```python
from build123d import *

# Parameters (mm, degrees)
SKETCH1_W              = 38.1
SKETCH1_H              = 76.2
BOSS_EXTRUDE1_DEPTH    = 2.54
F_1_0MM_DOWEL_HOLE1_D  = 19
M1_6_CLEARANCE_HOLE1_D = 1.8
M2_CLEARANCE_HOLE4_D   = 2.4
SKETCH15_R             = 3.749999993
BOSS_EXTRUDE2_DEPTH    = 10.000000066


with BuildPart() as part:
    # Sketch1 → Boss-Extrude1 (new body)
    with BuildSketch(Plane(origin=(0, 0, 0), x_dir=(1, 0, 0), z_dir=(0, 1, 0))):
        Rectangle(SKETCH1_W, SKETCH1_H)
    extrude(amount=BOSS_EXTRUDE1_DEPTH)

    # Ø1.0mm Dowel Hole1 (through all)
    with Locations(Plane(origin=(0, 2.54, 0), x_dir=(1, 0, 0), z_dir=(0, 1, 0))):
        with Locations((0, -13.000000035), (0, 13.000000035)):
            Hole(F_1_0MM_DOWEL_HOLE1_D / 2)

    # M1.6 Clearance Hole1 (through all)
    with Locations(Plane(origin=(0, 2.54, 0), x_dir=(1, 0, 0), z_dir=(0, 1, 0))):
        with Locations((8.750000026, 21.250000045), (8.750000026, -21.250000045), (-8.750000026, -21.250000045), (-8.750000026, 21.250000045)):
            Hole(M1_6_CLEARANCE_HOLE1_D / 2)

    # M2 Clearance Hole4 (through all)
    with Locations(Plane(origin=(0, 2.54, 0), x_dir=(1, 0, 0), z_dir=(0, 1, 0))):
        with Locations((-13.97, 33.02), (13.97, 33.02), (-13.97, -33.02), (13.97, -33.02)):
            Hole(M2_CLEARANCE_HOLE4_D / 2)

    # Sketch15 → Boss-Extrude2 (add)
    with BuildSketch(Plane(origin=(0, 2.54, 0), x_dir=(1, 0, 0), z_dir=(0, 1, 0))):
        with Locations((-13.97, -26.035)):
            Circle(SKETCH15_R)
        with Locations((13.97, -26.035)):
            Circle(SKETCH15_R)
    boss_extrude2 = extrude(amount=BOSS_EXTRUDE2_DEPTH)

    # Mirror1: Boss-Extrude2 across plane
    add(boss_extrude2.mirror(Plane.XY))


solid = part.part
```
Model file for the job. Use its own axes, mm. A direction names the side the tool comes from. Coordinates: 2 decimals unless noted, no trailing zeros. Order: outer loops, then holes, each group sorted by start corner. A loop starts at its lowest first (then second) coordinate and runs counter-clockwise, first axis right, second up. Notation, with made-up numbers: M 73,12.25 L 99,12.25 A12 cw 99,31.25 Z; hole C 49.5,-25 d10. An arc over 180 degrees is marked long. Answer as CSV lines item,"result".
(1) Band-saw the part on A-A, the plane x = 13.97. List the corners of the cut face in (y, z) (3 decimals), then the cut area to 3 significant figures.
Geometry says:
outline,"M 0,-38.1 L 2.54,-38.1 L 2.54,-34.22 L 0,-34.22 Z; M 0,-31.82 L 2.54,-31.82 L 2.54,-29.785 L 12.54,-29.785 L 12.54,-22.285 L 2.54,-22.285 L 2.54,22.285 L 12.54,22.285 L 12.54,29.785 L 2.54,29.785 L 2.54,31.82 L 0,31.82 Z; M 0,34.22 L 2.54,34.22 L 2.54,38.1 L 0,38.1 Z"
area,"331 mm2"
(2) Flat gauge pins, fed straight in: pin 1 (1.6 mm diameter, centred on x = 8.75, z = 21.25, fed in from +Y); pin 2 (4 mm diameter, centred on x = -13.97, z = -33.02, fed in from +Y). Where does each tip first touch, or does it go through?
Geometry says:
pin 1,"passes through"
pin 2,"stops at y = 2.54"
(3) Band-saw the part on B-B, the plane z = 33.02. List the corners of the cut face in (x, y).
Geometry says:
outline,"M -19.05,0 L -15.17,0 L -15.17,2.54 L -19.05,2.54 Z; M -12.77,0 L 12.77,0 L 12.77,2.54 L -12.77,2.54 Z; M 15.17,0 L 19.05,0 L 19.05,2.54 L 15.17,2.54 Z"
(4) Band-saw the part on C-C, the plane y = 1.25. State how many separate pieces and enclosed holes the cut face has, then the cut area to 3 significant figures.
Geometry says:
separate pieces,"1"
enclosed holes,"10"
area,"2,310 mm2"
(5) Band-saw the part on D-D, the plane z = -13. List the corners of the cut face in (x, y), then the cut area to 3 significant figures.
Geometry says:
outline,"M -19.05,0 L -9.5,0 L -9.5,2.54 L -19.05,2.54 Z; M 9.5,0 L 19.05,0 L 19.05,2.54 L 9.5,2.54 Z"
area,"48.5 mm2"
(6) 3-axis set-ups, long thin cutter, end or side, ignore diameter. For faces 1 (the flat face through (0, 2.54, -1)), 2 (the flat face through (0, 0, -1)): which of +Z, -Z, +X, -X, +Y, -Y reach the whole face in a straight line?
Geometry says:
face 1,"+Y"
face 2,"+Z, -Z, +X, -X, -Y"
(7) Pull direction X, two halves, no side cores. Call faces 3 (the flat face through (0, 1, 38.1)), 4 (the cylindrical face through (-9.061, 1.252, -15.854)), 5 (the flat face through (19.05, 1, 1)), 6 (the cylindrical face through (13.157, 7.47, -29.696)): +X half, -X half, draft (parallel to the pull), parting line (faces both ways), or undercut.
Geometry says:
face 3,"draft"
face 4,"undercut"
face 5,"+X half"
face 6,"undercut"
(8) Wall check: line 1 along X through (y, z) = (0.85, -33.02); line 2 along Z through (x, y) = (-13.97, 1.3); line 3 along Z through (x, y) = (3, 1.5). Give the ranges that are in metal, low to high.
Geometry says:
line 1,"x = -19.05 to -15.17, -12.77 to 12.77, 15.17 to 19.05"
line 2,"z = -38.1 to -34.22, -31.82 to 31.82, 34.22 to 38.1"
line 3,"z = -38.1 to -22.01, -3.99 to 3.99, 22.01 to 38.1"
